```python
from build123d import *

# Parameters (mm, degrees)
F0_W     = 120.626696
F0_H     = 83.924868
F0_R     = 6.75531
F0_R_2   = 6.692983
F1_DEPTH = 76.2
F2_R     = 26.889351
F3_DEPTH = 101.6
F5_DEPTH = 12.7
F7_DEPTH = 12.7


with BuildPart() as f1:
    # F0 (on Top) → F1 (new body)
    with BuildSketch(Plane.XY):
        Rectangle(F0_W, F0_H)
        with Locations((-47.834724, 0)):
            Circle(F0_R, mode=Mode.SUBTRACT)
        with Locations((48.568763, 0)):
            Circle(F0_R_2, mode=Mode.SUBTRACT)
    extrude(amount=F1_DEPTH)

    # F2 (on face) → F3 (cut)
    with BuildSketch(Plane.XZ.offset(41.962434)):
        with Locations((0, 76.2)):
            Circle(F2_R)
    extrude(amount=-F3_DEPTH, mode=Mode.SUBTRACT)

    # F4 (on face) → F5 (join)
    with BuildSketch(Plane.XZ.offset(41.962434)):
        with BuildLine():
            Line((-26.889351, 76.2), (-35.875045, 76.2))
            ThreePointArc((-35.875045, 76.2), (0, 40.324955), (35.875045, 76.2))
            Line((35.875045, 76.2), (26.889351, 76.2))
            ThreePointArc((26.889351, 76.2), (0, 49.310649), (-26.889351, 76.2))
        make_face()
    extrude(amount=F5_DEPTH)

    # F6 (on face) → F7 (join)
    with BuildSketch(Plane(origin=(0, 41.962434, 0), x_dir=(-1, 0, 0), z_dir=(0, 1, 0))):
        with BuildLine():
            Line((-26.889351, 76.2), (-37.436254, 76.2))
            ThreePointArc((-37.436254, 76.2), (0, 38.763746), (37.436254, 76.2))
            Line((37.436254, 76.2), (26.889351, 76.2))
            ThreePointArc((26.889351, 76.2), (0, 49.310649), (-26.889351, 76.2))
        make_face()
    extrude(amount=F7_DEPTH)


solid = f1.part
```
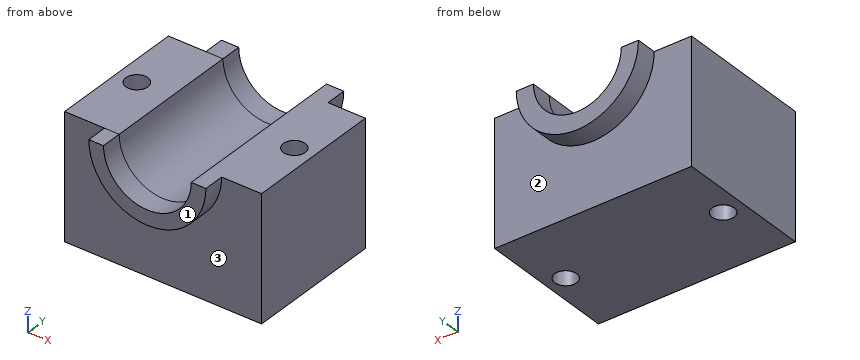
Design review of the part built by this model. Coordinates are the model's own, in mm. Face numbers are marked on the shaded views. A direction names the side the tool comes from. Coordinates: 2 decimals unless noted, no trailing zeros. Loops run counter-clockwise (first coordinate to the right, second up) from the corner with the lowest first, then second, coordinate; pieces in that order, holes last. Notation, with made-up numbers: (80.5, 36) -> (133.5, 36) arc R24 ccw to (133.5, 55) -> close; hole circle Ø11 at (70, 9). An arc over 180 degrees is marked (long way). Answer as a JSON object with one key per item and string values.
Q1. Take a section at D-D on y = -17.5. Give the boundary of the cut face in (x, z).
Answer block:
{"outline": "(-60.31, 0) -> (60.31, 0) -> (60.31, 76.2) -> (26.89, 76.2) arc R26.89 cw to (-26.89, 76.2) -> (-60.31, 76.2) -> close"}
Q2. Take a section at B-B on x = 0. Give the boundary of the cut face in (y, z).
Answer block:
{"outline": "(-54.66, 40.32) -> (-41.96, 40.32) -> (-41.96, 0) -> (41.96, 0) -> (41.96, 38.76) -> (54.66, 38.76) -> (54.66, 49.31) -> (-54.66, 49.31) -> close"}
Q3. Take a section at C-C on z = 42.5. Give the boundary of the cut face in (x, y).
Answer block:
{"outline": "(-60.31, -41.96) -> (-12.3, -41.96) -> (-12.3, -54.66) -> (12.3, -54.66) -> (12.3, -41.96) -> (60.31, -41.96) -> (60.31, 41.96) -> (16.3, 41.96) -> (16.3, 54.66) -> (-16.3, 54.66) -> (-16.3, 41.96) -> (-60.31, 41.96) -> close; hole circle Ø13.51 at (-47.83, 0); hole circle Ø13.39 at (48.57, 0)"}
Q4. To check wall thickness, follow L1, parallel to Y at x = -37, z = 55.5; L2, parallel to Y at x = -45, z = 15; L3, parallel to Y at x = -53, z = 12. State the ranges of each line that lie inside material, in increasing order.
Answer block:
{"L1": "y = -41.96 to 41.96", "L2": "y = -41.96 to -6.13, 6.13 to 41.96", "L3": "y = -41.96 to -4.35, 4.35 to 41.96"}
Q5. Take a section at A-A on y = 0. Give the boundary of the cut face in (x, z).
Answer block:
{"outline": "(-60.31, 0) -> (-54.59, 0) -> (-54.59, 76.2) -> (-60.31, 76.2) -> close; (-41.08, 0) -> (41.88, 0) -> (41.88, 76.2) -> (26.89, 76.2) arc R26.89 cw to (-26.89, 76.2) -> (-41.08, 76.2) -> close; (55.26, 0) -> (60.31, 0) -> (60.31, 76.2) -> (55.26, 76.2) -> close"}
Q6. Clearance check with flat-ended pins moving along their axes: pin 1 Ø12 at (x, z) = (-16.5, 68) entering from +Y; pin 2 Ø1 at (x, z) = (43, 65) entering from -Y; pin 3 Ø8 at (x, z) = (44, 34.5) entering from +Y. State where each tip first meets the part, or that it passes through.
Answer block:
{"pin 1": "passes through", "pin 2": "stops at y = -41.96", "pin 3": "stops at y = 41.96"}
Q7. Tool access review of the marked faces 1, 2 and 3: name each direction out of +Z, -Z, +X, -X, +Y, -Y from which nothing blocks a thin tool from reaching the whole face with its end or side.
Answer block:
{"face 1": "+Z, -Z, +X, -X, -Y", "face 2": "-Z, +Y", "face 3": "-Z, -Y"}
